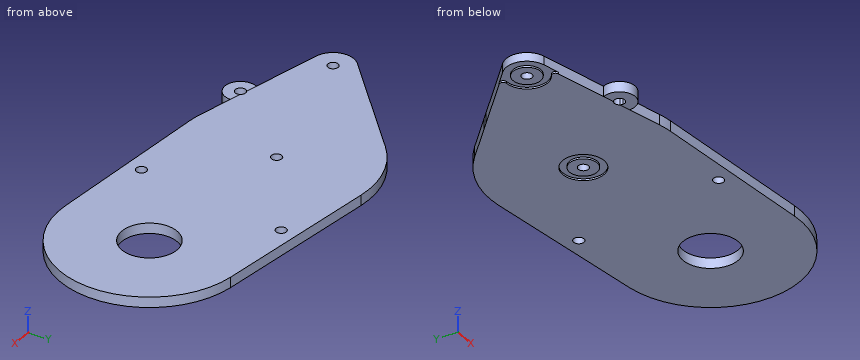
Autodesk Inventor part; units mm, degrees
ref_plane "YZ Plane" through (0, 0, 0) normal (1, 0, 0) x (0, 1, 0)
ref_plane "XZ Plane" through (0, 0, 0) normal (0, 1, 0) x (-1, 0, 0)
ref_plane "XY Plane" through (0, 0, 0) normal (0, 0, 1) x (1, 0, 0)
sketch "スケッチ1" plane through (0, 0, 0) normal (0, 0, 1) x (1, 0, 0)
  circle A0 centre (-27.1196, 80) radius 1.5
  circle A1 centre (-27.1196, 80) radius 6
  circle A2 centre (20.6799, 65) radius 1.5
  circle A3 centre (20.6799, 65) radius 6
  circle A4 centre (63.5417, 75.7941) radius 1.5
  circle A5 centre (-68.1796, 83.3936) radius 1.5
  circle A6 centre (-112.5, 70) radius 8.025
  circle A7 centre (112.5, 70) radius 8.025
  arc A8 (109.9686, 44.1235) -> (116.0788, 95.7525) centre (112.5, 70) ccw
  circle A9 centre (-94.9808, 96.6696) radius 4.5
  circle A10 centre (-94.9808, 96.6696) radius 1.5
  circle A11 centre (-83.1426, 57.4965) radius 1.5
  circle A12 centre (-83.1426, 57.4965) radius 4.5
  circle A13 centre (86.1018, 50.9798) radius 4.5
  circle A14 centre (86.1018, 50.9798) radius 1.5
  circle A15 centre (91.2708, 94.6568) radius 1.5
  circle A16 centre (91.2708, 94.6568) radius 4.5
  line L0 (-103.9107, 45.4598) -> (-60.251, 60.7411)
  line L1 (-118.9391, 95.19) -> (-74.1234, 106.646)
  line L2 (-55.9515, 104.0449) -> (-24.0626, 85.1628)
  line L3 (-24.9517, 74.4053) -> (-59.508, 61.015)
  line L4 (116.0788, 95.7525) -> (67.2581, 102.5371)
  line L5 (45.3001, 95.7) -> (16.6263, 69.4235)
  line L6 (19.2049, 59.1841) -> (56.904, 49.6227)
  line L7 (60.9129, 48.9224) -> (109.9686, 44.1235)
  arc A17 (-118.9391, 95.19) -> (-103.9107, 45.4598) centre (-112.5, 70) ccw
  arc A18 (-60.251, 60.7411) -> (-59.508, 61.015) centre (-68.1796, 83.3936) ccw
  arc A19 (-55.9515, 104.0449) -> (-74.1234, 106.646) centre (-68.1796, 83.3936) ccw
  arc A20 (56.904, 49.6227) -> (60.9129, 48.9224) centre (63.5417, 75.7941) ccw
  arc A21 (67.2581, 102.5371) -> (45.3001, 95.7) centre (63.5417, 75.7941) ccw
  point P0 (0, 0)
  point P1 (0, 0)
  point P2 (0, 0)
  dimension "d0" = 3
  dimension "d1" = 12
  dimension "d2" = 3
  dimension "d3" = 12
  dimension "d4" = 3
  dimension "d5" = 3
  dimension "d6" = 16.05
  dimension "d7" = 16.05
  dimension "d8" = 52
  dimension "d9" = 9
  dimension "d10" = 3
  dimension "d11" = 3
  dimension "d12" = 9
  dimension "d13" = 9
  dimension "d14" = 3
  dimension "d15" = 3
  dimension "d16" = 9
  dimension "d17" = 2.0367
  dimension "d18" = 2.0367
  dimension "d19" = 24
  dimension "d20" = 24
  dimension "d21" = 26
  dimension "d22" = 27
  dimension "d23" = 27
  dimension "d24" = 31.9091
  dimension "d25" = 31.9091
  dimension "d26" = 32.5367
  dimension "d27" = 32.5367
extrude "押し出し1" add sketch "スケッチ1" along normal blind 3 contours A3 | A13 | A16 | A3 L5 A21 L4 A8 L7 A20 L6
sketch "スケッチ2" plane through (0, 0, 3) normal (0, 0, 1) x (1, 0, 0)
  arc A0 (56.904, 49.6227) -> (60.9129, 48.9224) centre (63.5417, 75.7941) ccw
  line L0 (60.9129, 48.9224) -> (109.9686, 44.1235)
  arc A1 (109.9686, 44.1235) -> (116.0788, 95.7525) centre (112.5, 70) ccw
  line L1 (116.0788, 95.7525) -> (67.2581, 102.5371)
  arc A2 (67.2581, 102.5371) -> (45.3001, 95.7) centre (63.5417, 75.7941) ccw
  line L2 (45.3001, 95.7) -> (16.6263, 69.4235)
  arc A3 (16.6263, 69.4235) -> (19.2049, 59.1841) centre (20.6799, 65) ccw
  line L3 (19.2049, 59.1841) -> (56.904, 49.6227)
  circle A4 centre (91.2708, 94.6568) radius 1.5
  circle A5 centre (86.1018, 50.9798) radius 1.5
  circle A6 centre (112.5, 70) radius 8.025
  circle A7 centre (63.5417, 75.7941) radius 1.5
  circle A8 centre (20.6799, 65) radius 1.5
  circle A9 centre (63.5417, 75.7941) radius 27
  circle A10 centre (20.6799, 65) radius 21
  circle A11 centre (34.0051, 86.7414) radius 4.5
  circle A12 centre (34.0051, 86.7414) radius 1.5
  circle A13 centre (42.7132, 52.1631) radius 1.5
  circle A14 centre (42.7132, 52.1631) radius 4.5
  point P0 (0, 0)
  point P1 (38.7185, 54.235)
  point P2 (47.2124, 52.0807)
  point P3 (44.0259, 52.8889)
  point P4 (41.9051, 53.4268)
  point P5 (35.505, 86.7239)
  point P6 (37.9287, 88.9449)
  point P7 (31.4683, 83.0247)
  point P8 (33.892, 85.2457)
  dimension "d30" = 54
  dimension "d31" = 42
  dimension "d32" = 9
  dimension "d33" = 3
  dimension "d34" = 3
  dimension "d35" = 9
extrude "押し出し2" add sketch "スケッチ2" against normal blind 3 contours A14 L3 A13
sketch "スケッチ3" plane through (0, 0, 3) normal (0, 0, 1) x (1, 0, 0)
  line L0 (47.2124, 52.0807) -> (56.904, 49.6227)
  arc A0 (56.904, 49.6227) -> (60.9129, 48.9224) centre (63.5417, 75.7941) ccw
  line L1 (60.9129, 48.9224) -> (109.9686, 44.1235)
  arc A1 (109.9686, 44.1235) -> (116.0788, 95.7525) centre (112.5, 70) ccw
  line L2 (116.0788, 95.7525) -> (67.2581, 102.5371)
  arc A2 (67.2581, 102.5371) -> (45.3001, 95.7) centre (63.5417, 75.7941) ccw
  line L3 (45.3001, 95.7) -> (16.6263, 69.4235)
  arc A3 (16.6263, 69.4235) -> (19.2049, 59.1841) centre (20.6799, 65) ccw
  circle A4 centre (91.2708, 94.6568) radius 1.5
  circle A5 centre (86.1018, 50.9798) radius 1.5
  circle A6 centre (112.5, 70) radius 8.025
  circle A7 centre (63.5417, 75.7941) radius 1.5
  circle A8 centre (20.6799, 65) radius 1.5
  circle A9 centre (34.0051, 86.7414) radius 1.5
  circle A10 centre (42.7132, 52.1631) radius 1.5
  arc A11 (38.7185, 54.235) -> (47.2124, 52.0807) centre (42.7132, 52.1631) ccw
  line L4 (19.2049, 59.1841) -> (38.7185, 54.235)
  point P0 (0, 0)
  point P1 (41.9051, 53.4268)
  point P2 (44.0259, 52.8889)
  point P3 (35.505, 86.7239)
  point P4 (33.892, 85.2457)
  dimension "d38" = 3
  dimension "d39" = 3
extrude "押し出し3" cut sketch "スケッチ3" against normal blind 3 contours A9 L3 | A10 picked at (33.6626, 86.26)
sketch "スケッチ4" plane through (0, 0, 0) normal (0, 0, -1) x (-1, 0, 0)
  circle A0 centre (-63.5417, 75.7941) radius 1.5
  circle A1 centre (-20.6799, 65) radius 1.5
  circle A2 centre (-20.6799, 65) radius 6
  circle A3 centre (-20.6799, 65) radius 4
  circle A4 centre (-63.5417, 75.7941) radius 4
  circle A5 centre (-63.5417, 75.7941) radius 6
  point P0 (0, 0)
  dimension "d42" = 12
  dimension "d43" = 8
  dimension "d44" = 8
  dimension "d45" = 12
extrude "押し出し4" cut sketch "スケッチ4" against normal blind 0.5 contours A2 | A5
fillet "フィレット1" radius 1 2 edges at (19.2049, 59.1841, 0.25) (16.6263, 69.4235, 0.25)
properties part number "後脚ギアトレイン5.1" material "アルミニウム 7075"
Could you check a few things on this model? Use its own coordinates, in mm. Give positions to 0.01 mm unless a question says otherwise; leave off trailing zeros. Order: outer loops, then holes, each group sorted by start corner. A loop starts at its lowest first (then second) coordinate and runs counter-clockwise, first axis right, second up. Notation, with made-up numbers: (49, -34) - (55, -34) arc R14 ccw to (55, -26) - close; hole circle Ø11 at (74, 6). An arc over 180 degrees is marked (long way). One line per question, with ' | ' between items. Start each with the question number.
Item 1: I want a section at B-B on y = 65. Write out the boundary of the cut face in (x, z).
Item 2: I need wall thicknesses on probe 1 along X at (y, z) = (68.5, 0.25); probe 2 along Y at (x, z) = (107, 0.8); probe 3 along Y at (x, z) = (86, 0.4). Which ranges of each line are inside material? Lowest first, please. Write a range as [from, to].
Item 3: I want a section at D-D on x = 55. Write out the boundary of the cut face in (y, z).
Item 4: I want a section at C-C on z = 1.05. Give the number of separate pieces and of enclosed holes in the cut face, then the cut area to 3 significant figures.
Item 5: I'm going to push a flat-ended pin straight in: pin 1 Ø1 at (y, z) = (60.5, 1.5) entering from -X. Where does the tip first touch, or does it pass through?
Item 6: I want a section at A-A on x = 112.5. Write out the boundary of the cut face in (y, z) (3 decimals), then the cut area to 3 significant figures.
Verdict:
1) outline: (14.68, 0.5) - (16.68, 0.5) - (16.68, 0) - (19.18, 0) - (19.18, 3) - (14.68, 3) - close; (22.18, 0) - (24.68, 0) - (24.68, 0.5) - (26.68, 0.5) - (26.68, 0) - (106.22, 0) - (106.22, 3) - (22.18, 3) - close; (118.78, 0) - (138.01, 0) - (138.01, 3) - (118.78, 3) - close
2) probe 1: [18.74, 22.62], [25.55, 104.62], [120.38, 138.46] | probe 2: [44.41, 64.16], [75.84, 97.01] | probe 3: [46.47, 49.48], [52.48, 99.93]
3) outline: (50.11, 0) - (101.41, 0) - (101.41, 3) - (50.11, 3) - close
4) separate pieces: 1 | enclosed holes: 6 | area: 5,160 mm^2
5) pin 1: x = 16.21
6) outline: (44, 0) - (61.975, 0) - (61.975, 3) - (44, 3) - close; (78.025, 0) - (96.25, 0) - (96.25, 3) - (78.025, 3) - close | area: 109 mm^2
